For this review, take the finished solid that the model builds, in its own axes (mm). A direction names the side the tool comes from. Round coordinates to 2 decimals unless told otherwise and drop trailing zeros. Write each loop counter-clockwise with the first axis right and the second up, starting at its lowest first coordinate (ties: lowest second). Pieces come first, ordered by that corner, then holes. Notation, with made-up numbers: (33.5, -24) -> (57.5, -24) arc R15 cw to (57.5, 4) -> close; hole circle Ø2 at (55, 48.25). An arc over 180 degrees is marked (long way). Write each question's results on one line, items separated by ' | '. Start each with the question number.
Item 1: The part is to be moulded in two halves that separate along X. For faces 1 (the flat face through (13, 5, 10)), 2 (the flat face through (0, 15, 0)), 3 (the flat face through (20, 7, 0)), say which applies: +X half, -X half, draft (parallel to the pull), parting line (faces both ways), or undercut.
Item 2: Clearance check with flat-ended pins moving along their axes: pin 1 (1.2 mm diameter, centred on x = -14, z = -11, fed in from -Y); pin 2 (3.5 mm diameter, centred on x = -9, z = 6.5, fed in from +Y). State where each tip first meets the part, or that it passes through.
Item 3: Add section D-D (x = -9.5). State the section outline as (y, z) points.
Item 4: Tool access review of faces 4 (the cylindrical face through (-15.286, 2.465, -9.566)), 5 (the cylindrical face through (-5.9, 5.5, 9.1)), 6 (the cylindrical face through (-6.483, 8.028, 11.055)): name each direction out of +Z, -Z, +X, -X, +Y, -Y from which nothing blocks a thin tool from reaching the whole face with its end or side.
Item 5: Add section C-C (z = 10.5). State the section outline as (x, y) points, plus the area to 3 significant figures.
Item 6: To check wall thickness, follow line 1 along X through (y, z) = (3.45, 10); line 2 along Y through (x, z) = (10.5, -9.25); line 3 along Y through (x, z) = (12.5, 10.5). State the ranges of each line that lie inside material, in increasing order.
Item 7: Add section A-A (x = 7.5). State the section outline as (y, z) points, plus the area to 3 significant figures.
Item 8: Add section B-B (y = 11.75). State the section outline as (x, z) points (3 decimals).
from build123d import *

# Parameters (mm, degrees)
SKETCH1_W               = 40
SKETCH1_H               = 30
BOSS_EXTRUDE1_DEPTH     = 10
SKETCH2_R               = 2
CUT_EXTRUDE1_DEPTH      = 5
SKETCH3_R               = 4.8125
CUT_EXTRUDE2_DEPTH      = 4
SKETCH5_W               = 40
SKETCH5_H               = 30
BOSS_EXTRUDE2_DEPTH     = 5
CUT_EXTRUDE3_DEPTH      = 27.570660511
CUT_EXTRUDE3_DEPTH_BACK = 1
SKETCH4_R               = 3.325


with BuildPart() as part:
    # Sketch1 → Boss-Extrude1 (new body)
    with BuildSketch(Plane(origin=(0, 0, 0), x_dir=(1, 0, 0), z_dir=(0, 1, 0))):
        Rectangle(SKETCH1_W, SKETCH1_H)
    extrude(amount=BOSS_EXTRUDE1_DEPTH)

    # Sketch2 → Cut-Extrude1 (cut)
    with BuildSketch(Plane(origin=(0, 0, 0), x_dir=(-1, 0, 0), z_dir=(0, -1, 0))):
        with Locations(Location((-13.333333333, -10, 0), (0, 0, 90))):
            Circle(SKETCH2_R)
        with Locations(Location((13.333333333, -10, 0), (0, 0, 270))):
            Circle(SKETCH2_R)
        with Locations(Location((-13.333333333, 10, 0), (0, 0, 270))):
            Circle(SKETCH2_R)
        with Locations(Location((13.333333333, 10, 0), (0, 0, 90))):
            Circle(SKETCH2_R)
    extrude(amount=-CUT_EXTRUDE1_DEPTH, mode=Mode.SUBTRACT)

    # Sketch3 → Cut-Extrude2 (cut)
    with BuildSketch(Plane(origin=(0, 10, 0), x_dir=(1, 0, 0), z_dir=(0, 1, 0))):
        with Locations(Location((-7.9286, -6.465, 0), (0, 0, 270))):
            Circle(SKETCH3_R)
        with Locations(Location((7.5, 6.4636, 0), (0, 0, 270))):
            Circle(SKETCH3_R)
    extrude(amount=-CUT_EXTRUDE2_DEPTH, mode=Mode.SUBTRACT)

    # Sketch5 → Boss-Extrude2 (add)
    with BuildSketch(Plane(origin=(0, 10, 0), x_dir=(1, 0, 0), z_dir=(0, 1, 0))):
        Rectangle(SKETCH5_W, SKETCH5_H)
    extrude(amount=BOSS_EXTRUDE2_DEPTH)

    # Sketch4 → Cut-Extrude3 (cut, two sides: drawn at the far end of the back side and taken through both)
    with BuildSketch(Plane(origin=(0, 6, 0), x_dir=(1, 0, 0), z_dir=(0, 1, 0)).offset(-CUT_EXTRUDE3_DEPTH_BACK)):
        with Locations(Location((-7.9286, -6.465, 0), (0, 0, 90))):
            Circle(SKETCH4_R)
        with Locations(Location((7.5, 6.4636, 0), (0, 0, 90))):
            Circle(SKETCH4_R)
    extrude(amount=CUT_EXTRUDE3_DEPTH + CUT_EXTRUDE3_DEPTH_BACK, mode=Mode.SUBTRACT)


solid = part.part
Responses:
1) face 1: undercut | face 2: draft | face 3: +X half
2) pin 1: stops at y = 5 | pin 2: stops at y = 5
3) outline: (0, -15) -> (15, -15) -> (15, 3.53) -> (10, 3.53) -> (10, 1.92) -> (6, 1.92) -> (6, 3.53) -> (5, 3.53) -> (5, 9.4) -> (6, 9.4) -> (6, 11.01) -> (10, 11.01) -> (10, 9.4) -> (15, 9.4) -> (15, 15) -> (0, 15) -> close
4) face 4: -Y | face 5: +Y | face 6: none
5) outline: (-20, 0) -> (-15.27, 0) -> (-15.27, 5) -> (-11.4, 5) -> (-11.4, 0) -> (11.4, 0) -> (11.4, 5) -> (15.27, 5) -> (15.27, 0) -> (20, 0) -> (20, 15) -> (-20, 15) -> close; hole (-10.55, 6) -> (-5.31, 6) -> (-5.31, 10) -> (-10.55, 10) -> close | area: 540 mm^2
6) line 1: x = -20 to -15.33, -11.33 to 11.33, 15.33 to 20 | line 2: y = 0 to 6, 10 to 15 | line 3: y = 5 to 15
7) outline: (0, -15) -> (15, -15) -> (15, -9.79) -> (10, -9.79) -> (10, -11.28) -> (6, -11.28) -> (6, -9.79) -> (5, -9.79) -> (5, -3.14) -> (6, -3.14) -> (6, -1.65) -> (10, -1.65) -> (10, -3.14) -> (15, -3.14) -> (15, 15) -> (0, 15) -> close | area: 372 mm^2
8) outline: (-20, -15) -> (20, -15) -> (20, 15) -> (-20, 15) -> close; hole circle Ø6.65 at (-7.929, 6.465); hole circle Ø6.65 at (7.5, -6.464)
